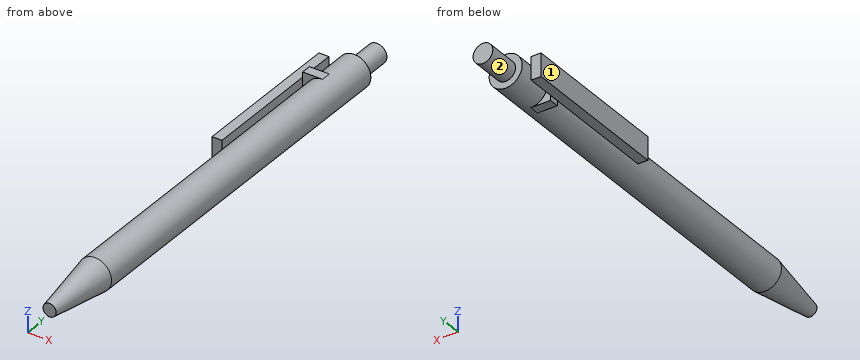
from build123d import *

# Parameters (mm, degrees)
ESBO_O3_R                = 5
RESSALTO_EXTRUS_O1_DEPTH = 100
RESSALTO_EXTRUS_O2_DEPTH = 3
ESBO_O5_W                = 7
ESBO_O5_H                = 47
RESSALTO_EXTRUS_O3_DEPTH = 3
ESBO_O6_R                = 5
RESSALTO_EXTRUS_O4_DEPTH = 11
ESBO_O7_R                = 3
RESSALTO_EXTRUS_O5_DEPTH = 10


with BuildPart() as part:
    # Esboço2 → Revolução1 (revolve)
    with BuildSketch(Plane.XY):
        Polygon((2, 0), (5, 20), (0, 20), (0, 0), align=None)
    revolve(axis=Axis((0, 22.732303323, 0), (0, -1, 0)))

    # Esboço3 → Ressalto-extrusão1 (add)
    with BuildSketch(Plane(origin=(0, 20, 0), x_dir=(1, 0, 0), z_dir=(0, 1, 0))):
        Circle(ESBO_O3_R)
    extrude(amount=RESSALTO_EXTRUS_O1_DEPTH)

    # Esboço4 → Ressalto-extrusão2 (add)
    with BuildSketch(Plane(origin=(0, 120, 0), x_dir=(1, 0, 0), z_dir=(0, 1, 0))):
        with BuildLine():
            Line((-6, 5), (0, 5))
            ThreePointArc((0, 5), (5, 0), (0, -5))
            Line((0, -5), (-6, -5))
            Line((-6, -5), (-6, 5))
        make_face()
    extrude(amount=RESSALTO_EXTRUS_O2_DEPTH)

    # Esboço5 → Ressalto-extrusão3 (add)
    with BuildSketch(Plane.ZY.offset(6)):
        with Locations((0, 108)):
            Rectangle(ESBO_O5_W, ESBO_O5_H)
    extrude(amount=RESSALTO_EXTRUS_O3_DEPTH)

    # Esboço6 → Ressalto-extrusão4 (add)
    with BuildSketch(Plane(origin=(0, 123, 0), x_dir=(1, 0, 0), z_dir=(0, 1, 0))):
        Circle(ESBO_O6_R)
    extrude(amount=RESSALTO_EXTRUS_O4_DEPTH)

    # Esboço7 → Ressalto-extrusão5 (add)
    with BuildSketch(Plane(origin=(0, 134, 0), x_dir=(1, 0, 0), z_dir=(0, 1, 0))):
        Circle(ESBO_O7_R)
    extrude(amount=RESSALTO_EXTRUS_O5_DEPTH)


solid = part.part
Part model, mm, in its own coordinate system. Face numbers are marked on the shaded views. A direction names the side the tool comes from. Coordinates: 2 decimals unless noted, no trailing zeros. Order: outer loops, then holes, each group sorted by start corner. A loop starts at its lowest first (then second) coordinate and runs counter-clockwise, first axis right, second up.
(1) Slice it at B-B, the plane z = 0. Write the cut outline in (x, y), and give its area (3 significant figures).
Check sheet entries:
outline: (-9, 84.5) - (-6, 84.5) - (-6, 120) - (-5, 120) - (-5, 20) - (-2, 0) - (2, 0) - (5, 20) - (5, 134) - (3, 134) - (3, 144) - (-3, 144) - (-3, 134) - (-5, 134) - (-5, 123) - (-6, 123) - (-6, 131.5) - (-9, 131.5) - close
area: 1,480 mm2
(2) Probe L1, parallel to Z at x = 0.25, y = 120; L2, parallel to Y at x = -5, z = -4.25; L3, parallel to X at y = 78, z = -4. List the from-to ranges inside material, lowest first.
Check sheet entries:
L1: z = -4.99 to 4.99
L2: y = 120 to 123
L3: x = -3 to 3
(3) Pin check, flat tips, straight feed: pin 1 Ø6 at (x, y) = (-3, 64) entering from +Z; pin 2 Ø3.5 at (x, z) = (-7, -1.5) entering from +Y; pin 3 Ø2.5 at (x, y) = (-7, 101.5) entering from -Z; pin 4 Ø1.5 at (x, z) = (-7.5, 1) entering from -Y. Stop position of each tip, or through.
Check sheet entries:
pin 1: stops at z = 5
pin 2: stops at y = 131.5
pin 3: stops at z = -3.5
pin 4: stops at y = 84.5
(4) Slice it at A-A, the plane y = 95.5. Write the cut outline in (x, z).
Check sheet entries:
outline: (-9, -3.5) - (-6, -3.5) - (-6, 3.5) - (-9, 3.5) - close; circle Ø10 at (0, 0)
(5) Slice it at C-C, the plane y = 53. Write the cut outline in (x, z), and give its area (3 significant figures).
Check sheet entries:
outline: circle Ø10 at (0, 0)
area: 78.5 mm2
(6) Tool access for the marked faces 1 and 2: list every direction of +Z, -Z, +X, -X, +Y, -Y with a clear straight run to the whole face (end or side of a thin tool).
Check sheet entries:
face 1: +Z, -Z, -X, +Y, -Y
face 2: +Y
